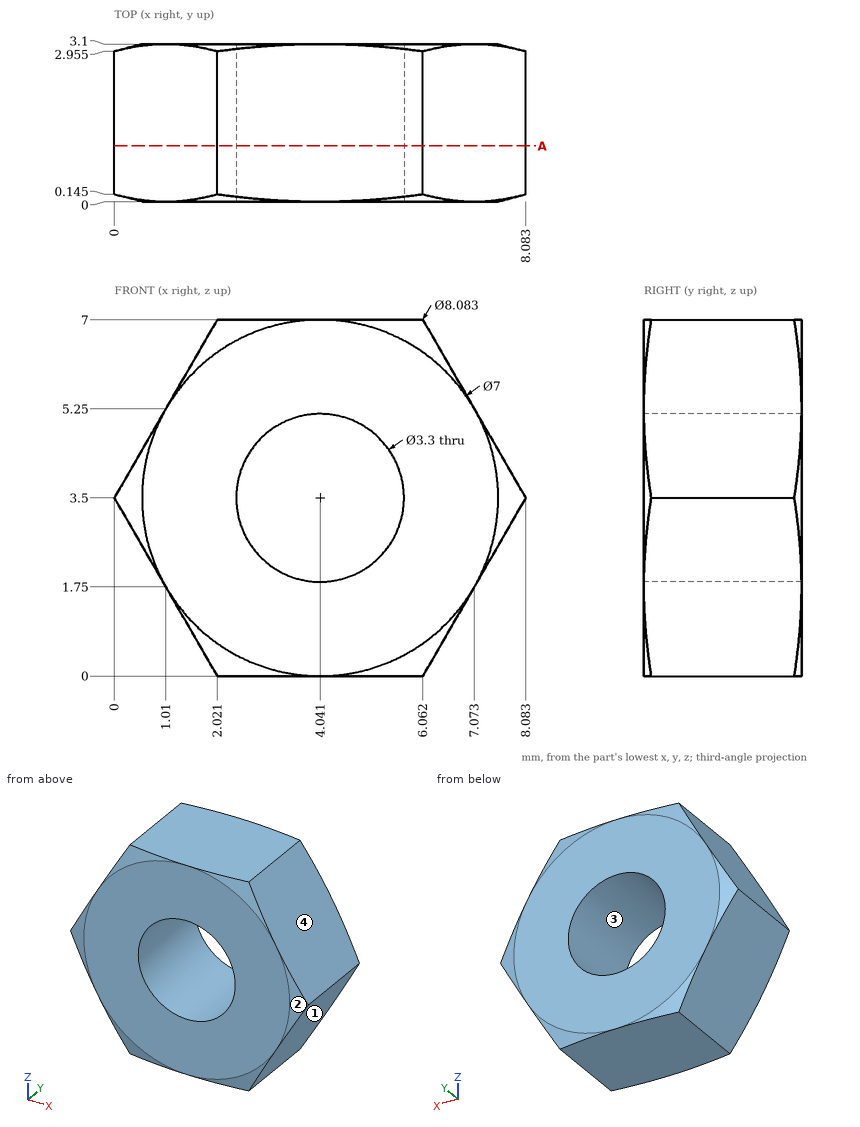
Can you work these out from the drawing? Everything is in mm from the part's minimum corner. Give positions to 0.01 mm unless a question says otherwise; leave off trailing zeros. Order: outer loops, then holes, each group sorted by start corner. A loop starts at its lowest first (then second) coordinate and runs counter-clockwise, first axis right, second up.
Item 1: If we section it at A-A, the plane y = 1.1: Write out the boundary of the cut face in (x, z).
Item 2: I need wall thicknesses on line 1 (X direction, y = 0.2, z = 4.5) (1 decimal); line 2 (Z direction, x = 3, y = 1.55); line 3 (X direction, y = 2.9, z = 4) (1 decimal). Which ranges of each line are inside material? Lowest first, please.
Item 3: If we mould it in two halves opening along Z, with no side actions, what happens to the marked faces 1, 2, 3 and 4? For each: pulls with the +Z half, pulls with the -Z half, needs draft (parallel to the pull), parting line crosses it, or undercut.
Item 4: I'm going to push a flat-ended pin straight in: pin 1 (1.5 mm diameter, centred on y = 2.5, z = 4.5, fed in from +X). Where does the tip first touch, or does it pass through?
Values:
1. outline: (0, 3.5) - (2.02, 0) - (6.06, 0) - (8.08, 3.5) - (6.06, 7) - (2.02, 7) - close; hole circle Ø3.3 at (4.04, 3.5)
2. line 1: x = 0.6 to 2.7, 5.4 to 7.5
2. line 2: z = 0 to 2.22, 4.78 to 7
2. line 3: x = 0.3 to 2.5, 5.6 to 7.8
3. face 1: pulls with the -Z half
3. face 2: parting line crosses it
3. face 3: undercut
3. face 4: pulls with the +Z half
4. pin 1: stops at x = 7.94
